from build123d import *

# Parameters (mm, degrees)
EXTRUDE_1_DEPTH         = 180
CUT_EXTRUDE_START       = -1.25
CUT_EXTRUDE_1_OUTLINE_W = 200.912361756
CUT_EXTRUDE_1_OUTLINE_H = 41.35790762
CUT_EXTRUDE_1_OUTLINE_R = 4
CUT_EXTRUDE_1_DEPTH     = 2.5


# Read off the part's stored shape, not the designer's step: 切除-拉伸1
with BuildPart() as part:
    # 草图2 → 凸台-拉伸1 (new body)
    with BuildSketch(Plane(origin=(0, 0, 0), x_dir=(0, 0, -1), z_dir=(1, 0, 0))):
        with BuildLine():
            Line((4.841229183, 1.25), (0, 1.25))
            Line((0, 1.25), (0, -1.25))
            Line((0, -1.25), (4.841229183, -1.25))
            ThreePointArc((4.841229183, -1.25), (4.960148481, -0.630021462), (5, 0))
            ThreePointArc((5, 0), (4.960148481, 0.630021462), (4.841229183, 1.25))
        make_face()
        with BuildLine():
            Line((0, -1.25), (0, 1.25))
            Line((0, 1.25), (-4.841229183, 1.25))
            ThreePointArc((-4.841229183, 1.25), (-5, 0), (-4.841229183, -1.25))
            Line((-4.841229183, -1.25), (0, -1.25))
        make_face()
    extrude(amount=EXTRUDE_1_DEPTH)

    # 切除-拉伸1 outline → 切除-拉伸1 (cut)
    # profile 1 of 2: a face of its own
    with BuildSketch(Plane(origin=(0, 0, 0), x_dir=(1, 0, 0), z_dir=(0, 1, 0)).offset(CUT_EXTRUDE_START)):
        with Locations((92.35420838, -2.241239646)):
            Rectangle(CUT_EXTRUDE_1_OUTLINE_W, CUT_EXTRUDE_1_OUTLINE_H)
        with BuildLine():
            Line((90, 5), (90, -5))
            Line((90, -5), (13.074176, -5))
            ThreePointArc((13.074176, -5), (8.074176, 0), (13.074176, 5))
            Line((13.074176, 5), (90, 5))
        make_face(mode=Mode.SUBTRACT)
    # profile 2 of 2: a face of its own
    with BuildSketch(Plane(origin=(0, 0, 0), x_dir=(1, 0, 0), z_dir=(0, 1, 0)).offset(CUT_EXTRUDE_START)):
        with Locations((13.074176, 0)):
            Circle(CUT_EXTRUDE_1_OUTLINE_R)
    extrude(amount=CUT_EXTRUDE_1_DEPTH, mode=Mode.SUBTRACT)

    # 草图4 → 切除-旋转3 (revolve, cut)
    with BuildSketch(Plane(origin=(0, 0, 0), x_dir=(1, 0, 0), z_dir=(0, 1, 0))):
        with BuildLine():
            Line((17.656751695, 2), (93.188618098, 2))
            Line((93.188618098, 2), (93.188618098, 5))
            Line((93.188618098, 5), (13.074176, 5))
            ThreePointArc((13.074176, 5), (15.812788788, 4.183300133), (17.656751695, 2))
        make_face()
        with BuildLine():
            Line((93.188618098, -4.841229183), (93.188618098, -2))
            Line((93.188618098, -2), (17.656751695, -2))
            ThreePointArc((17.656751695, -2), (16.318074985, -3.804880993), (14.324176, -4.841229183))
            Line((14.324176, -4.841229183), (93.188618098, -4.841229183))
        make_face()
    revolve(axis=Axis((18.074176, 0, 0), (1, 0, 0)), mode=Mode.SUBTRACT)

    # 镜向1: part across plane


with BuildPart() as part_1:
    add(part.part)
    add(part.part.mirror(Plane(origin=(90, 170, 0), x_dir=(0, 0, 1), z_dir=(1, 0, 0))))


solid = part_1.part
Could you check a few things on this model? Use its own coordinates, in mm. A direction names the side the tool comes from. Coordinates: 2 decimals unless noted, no trailing zeros. Loops run counter-clockwise (first coordinate to the right, second up) from the corner with the lowest first, then second, coordinate; pieces in that order, holes last.
1. Imagine slicing it at C-C (x = 88). Please give me the cut outline in (y, z), and give its area (3 significant figures).
2. I need wall thicknesses on L1, parallel to X at y = 0.65, z = -0.25; L2, parallel to X at y = 0.2, z = -3; L3, parallel to X at y = 0.5, z = -3. Which ranges of each line are inside material? Lowest first, please.
3. Imagine slicing it at A-A (z = 0). Please give me the cut outline in (x, y), and give its area (3 significant figures).
4. For P1, Ø1.5, axis at x = 50.5, y = -0.5, coming from the +Z side; P2, Ø1, axis at y = 0.5, z = -2, coming from the +X side, each with a flat end and sliding along its axis, tell me the tip position at first contact or that it passes through.
5. We'd pull the mould along X, two halves only. Please class faces 3 (the face through (8.075, -0.018, 0.11)), 4 (the face through (90, -1.25, 0)), 5 (the face through (89, 0, 2)): released by +X, released by -X, zero draft, split by the parting line, or undercut.
6. Imagine slicing it at B-B (y = -0.6). Please give me the cut outline in (x, z), and give its area (3 significant figures).
7. For faces 1 (the face through (89, 0, -2)), 2 (the face through (90, 1.25, 0)), which set-ups out of +Z, -Z, +X, -X, +Y, -Y let a thin tool reach every point of the face, with its end or its side?
Computed values:
1. outline: (-1.25, -1.56) arc R2 ccw to (1.25, -1.56) - (1.25, 1.56) arc R2 ccw to (-1.25, 1.56) - close
1. area: 9.30 mm2
2. L1: x = 8.08 to 9.08, 17.07 to 162.93, 170.92 to 171.92
2. L2: x = 9.07 to 10.43, 15.72 to 17.07, 162.93 to 164.28, 169.57 to 170.93
2. L3: x = 9.07 to 10.43, 15.72 to 17.04, 162.96 to 164.28, 169.57 to 170.93
3. outline: (8.07, -1.25) - (9.07, -1.25) - (9.07, 1.25) - (8.07, 1.25) - close; (17.07, -1.25) - (162.93, -1.25) - (162.93, 1.25) - (17.07, 1.25) - close; (170.93, -1.25) - (171.93, -1.25) - (171.93, 1.25) - (170.93, 1.25) - close
3. area: 370 mm2
4. P1: stops at z = 2
4. P2: stops at x = 171.7
5. face 3: released by -X
5. face 4: zero draft
5. face 5: undercut
6. outline: (12.47, -4.96) - (13.07, -4.96) arc R4.96 ccw to (17.66, -1.91) - (162.34, -1.91) arc R4.96 ccw to (166.93, -4.96) - (167.53, -4.96) arc R5 ccw to (167.53, 4.96) - (166.93, 4.96) arc R4.96 ccw to (162.34, 1.91) - (17.66, 1.91) arc R4.96 ccw to (13.07, 4.96) - (12.47, 4.96) arc R5 ccw to start; hole circle Ø8 at (13.07, 0); hole circle Ø8 at (166.93, 0)
6. area: 605 mm2
7. face 1: -Z
7. face 2: +Z, -Z, +X, -X, +Y
